The model under review builds one solid part; all positions refer to its coordinate system, in mm. Face numbers are marked on the shaded views. Round coordinates to 2 decimals unless told otherwise and drop trailing zeros. Order: outer loops, then holes, each group sorted by start corner. A loop starts at its lowest first (then second) coordinate and runs counter-clockwise, first axis right, second up. Notation, with made-up numbers: M -19.75,43 L 32.25,43 A16 cw 32.25,62 Z; hole C 67,10 d6. An arc over 180 degrees is marked long. Answer as a JSON object with one key per item and string values. Group by question number.
1. Add section B-B on z = -14.5. State the section outline as (x, y) points, and give its area (3 significant figures).
2. Clearance check with flat-ended pins moving along their axes: P1, Ø1.5, axis at x = -2, z = -12, coming from the -Y side; P2, Ø3, axis at y = -1, z = -4, coming from the +X side; P3, Ø2, axis at x = 1, z = -17, coming from the +Y side. State where each tip first meets the part, or that it passes through.
3. To check wall thickness, follow probe 1 along Z at (x, y) = (-0.2, -0.05); probe 2 along Z at (x, y) = (-0.75, -1.6); probe 3 along X at (y, z) = (0.65, -1). State the ranges of each line that lie inside material, in increasing order. Write a range as [from, to].
4. Mouldability with a two-part tool opening along Y and no side actions: class the marked faces 1, 2 and 3 as released by +Y, released by -Y, zero draft, split by the parting line, or undercut.
5. Add section A-A on x = 0. State the section outline as (y, z) points, and give its area (3 significant figures).
Autodesk Inventor part; units mm, degrees
ref_plane "YZ Plane" through (0, 0, 0) normal (1, 0, 0) x (0, 1, 0)
ref_plane "XZ Plane" through (0, 0, 0) normal (0, 1, 0) x (-1, 0, 0)
ref_plane "XY Plane" through (0, 0, 0) normal (0, 0, 1) x (1, 0, 0)
sketch "Sketch3" plane through (0, 0, 0) normal (0, 0, 1) x (1, 0, 0)
  circle A0 centre (0, 0) radius 1.5
  dimension "Diameter" = 3
extrude "Extrusion1" add sketch "Sketch3" against normal blind 20
sketch "Sketch4" plane through (0, 0, 0) normal (0, 0, 1) x (1, 0, 0)
  circle A0 centre (0, 0) radius 1.5
  circle A1 centre (0, 0) radius 2.75
  dimension "Head_Diameter" = 5.5
extrude "Extrusion2" add sketch "Sketch4" along normal blind 3 contours A0 | A1
sketch "Sketch5" plane through (0, 0, 3) normal (0, 0, 1) x (1, 0, 0)
  circle A0 centre (0, 0) radius 2.75
  line L0 (1.4434, 0) -> (0.7217, -1.25)
  line L1 (0.7217, -1.25) -> (-0.7217, -1.25)
  line L2 (-0.7217, -1.25) -> (-1.4434, 0)
  line L3 (-1.4434, 0) -> (-0.7217, 1.25)
  line L4 (-0.7217, 1.25) -> (0.7217, 1.25)
  line L5 (0.7217, 1.25) -> (1.4434, 0)
  line L6 (0, 0) -> (1.4434, 0) construction
  dimension "Hex_Width" = 2.5
extrude "Extrusion3" cut sketch "Sketch5" against normal blind 1.5 contours L0 L1 L2 L3 L4 L5
thread "Thread1"
chamfer "Chamfer1" distance 0.3 angle 45 1 edges at (-2.75, 0, 3)
chamfer "Chamfer2" distance 0.15 angle 45 1 edges at (-1.5, 0, -20)
equation "\"d14\" = 0.5 * Chamfer"
properties part number "SCREW,SOCKET-HD,P,12_9,M03X0_5X20MM" material "Steel, MS"
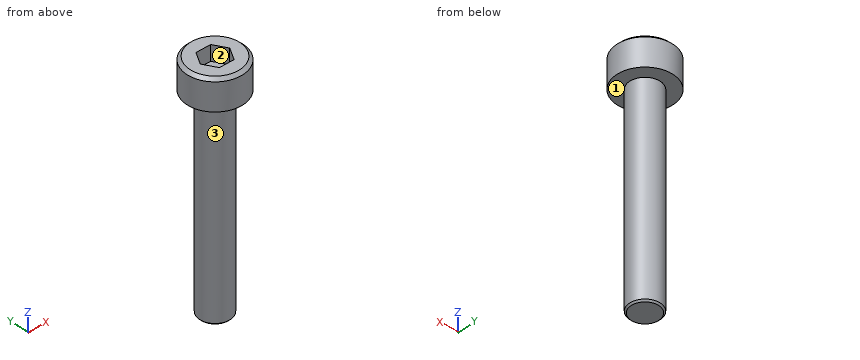
Recorded:
{
 "1": {"outline": "C 0,0 d3", "area": "7.07 mm²"},
 "2": {"P1": "stops at y = -0.83", "P2": "stops at x = 1.5", "P3": "stops at y = 1.5"},
 "3": {"probe 1": "z = [-20, 1.5]", "probe 2": "z = [0, 3]", "probe 3": "x = [-1.35, 1.35]"},
 "4": {"face 1": "zero draft", "face 2": "undercut", "face 3": "split by the parting line"},
 "5": {"outline": "M -2.75,0 L -1.5,0 L -1.5,-19.85 L -1.35,-20 L 1.35,-20 L 1.5,-19.85 L 1.5,0 L 2.75,0 L 2.75,2.7 L 2.45,3 L 1.25,3 L 1.25,1.5 L -1.25,1.5 L -1.25,3 L -2.45,3 L -2.75,2.7 Z", "area": "72.6 mm²"}
}
